The listing builds one solid part. Answer for the finished solid, in the listing's coordinates (mm). Face numbers are marked on the shaded views. A direction names the side the tool comes from. Coordinates: 2 decimals unless noted, no trailing zeros. Order: outer loops, then holes, each group sorted by start corner. A loop starts at its lowest first (then second) coordinate and runs counter-clockwise, first axis right, second up. Notation, with made-up numbers: (46, 13) -> (93, 13) arc R22 ccw to (93, 37) -> close; hole circle Ø5 at (25.25, -10.75). An arc over 180 degrees is marked (long way). Write each question's results on one line, items separated by ' | '. Start each with the question number.
(1) The part is cut by section D-D, the plane y = -47. Give the vertices of the cut face in (x, z), then the cut area to 3 significant figures.
(2) Determine the mould class of the marked faces 4, 5, 6 and 7 for opening direction Y: +Y half, -Y half, draft (parallel to the pull), parting line (faces both ways), or undercut.
(3) The part is cut by section B-B, the plane x = 73. Give the vertices of the cut face in (y, z), then the cut area to 3 significant figures.
(4) Given pin 1 (1.5 mm diameter, centred on x = 68, z = -24.5, fed in from +Y), flat-ended and moving along its own axis, determine where the tip first touches the part or whether it passes through.
(5) A tool of negligible diameter and unlimited length cuts with its end or side. For the marked faces 1, 2 and 3, from which of +Z, -Z, +X, -X, +Y, -Y can it reach the whole face along a straight path? Write none if from no direction.
(6) The part is cut by section A-A, the plane z = 17.5. Give the vertices of the cut face in (x, y).
(7) Straight lines are drawn through the part: L1, parallel to Y at x = -40.5, z = -9; L2, parallel to Y at x = -65, z = 15; L3, parallel to Z at x = 1, y = -57.5. For each, find the intervals that lie inside material, in ascending order.
(8) The part is cut by section C-C, the plane z = 2. Give the vertices of the cut face in (x, y), then the cut area to 3 significant figures.
```python
from build123d import *

# Parameters (mm, degrees)
F0_W      = 180.589676
F0_H      = 76.531302
F1_DEPTH  = 127
F4_DEPTH  = 127.001
F6_DEPTH  = 25.4
F8_DEPTH  = 25.4
F9_R      = 10.785345
F9_R_2    = 11.594885
F10_DEPTH = 25.4


with BuildPart() as f1:
    # F0 (on Front) → F1 (new body)
    with BuildSketch(Plane.XZ):
        with Locations((-1.058735, -6.049903)):
            Rectangle(F0_W, F0_H)
    extrude(amount=F1_DEPTH)

    # F2 (on face) → F4 (cut, through all)
    with BuildSketch(Plane.XZ.offset(127)):
        with BuildLine():
            Line((31.005763, 32.215748), (-31.913254, 32.215748))
            ThreePointArc((-31.913254, 32.215748), (-0.453746, 5.58325), (31.005763, 32.215748))
        make_face()
    extrude(amount=-F4_DEPTH, mode=Mode.SUBTRACT)

    # F3 (on face) → F6 (join)
    with BuildSketch(Plane.XZ.offset(127)):
        with BuildLine():
            ThreePointArc((31.005763, 32.215748), (-0.453746, 5.58325), (-31.913254, 32.215748))
            Line((-31.913254, 32.215748), (-40.383123, 32.215748))
            ThreePointArc((-40.383123, 32.215748), (-2e-06, -2.234087), (40.383119, 32.215748))
            Line((40.383119, 32.215748), (31.005763, 32.215748))
        make_face()
    extrude(amount=F6_DEPTH)

    # F7 (on face) → F8 (join)
    with BuildSketch(Plane(origin=(0, 0, 0), x_dir=(-1, 0, 0), z_dir=(0, 1, 0))):
        with BuildLine():
            Line((-31.005763, 32.215748), (-38.87064, 32.215748))
            ThreePointArc((-38.87064, 32.215748), (1.058737, -1.02799), (40.988114, 32.215748))
            Line((40.988114, 32.215748), (31.913254, 32.215748))
            ThreePointArc((31.913254, 32.215748), (0.453746, 5.58325), (-31.005763, 32.215748))
        make_face()
    extrude(amount=F8_DEPTH)

    # F9 (on face) → F10 (cut)
    with BuildSketch(Plane.XY.offset(32.215748)):
        with Locations((-63.675255, -62.828988)):
            Circle(F9_R)
        with Locations((64.280249, -62.828988)):
            Circle(F9_R_2)
    extrude(amount=-F10_DEPTH, mode=Mode.SUBTRACT)


solid = f1.part
```
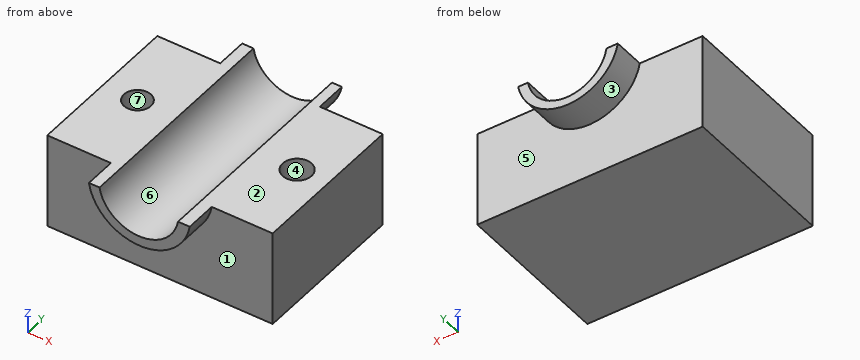
Established:
1) outline: (-91.35, -44.32) -> (89.24, -44.32) -> (89.24, 32.22) -> (31.01, 32.22) arc R31.9 cw to (-31.91, 32.22) -> (-91.35, 32.22) -> close | area: 12,600 mm^2
2) face 4: undercut | face 5: +Y half | face 6: draft | face 7: undercut
3) outline: (-127, -44.32) -> (0, -44.32) -> (0, 32.22) -> (-55.19, 32.22) -> (-55.19, 6.82) -> (-70.47, 6.82) -> (-70.47, 32.22) -> (-127, 32.22) -> close | area: 9,330 mm^2
4) pin 1: stops at y = 0
5) face 1: -Z, -Y | face 2: +Z, +X, -X, +Y, -Y | face 3: -Z, +Y
6) outline: (-91.35, -127) -> (-34.99, -127) -> (-34.99, -152.4) -> (-25.32, -152.4) -> (-25.32, 25.4) -> (-35.14, 25.4) -> (-35.14, 0) -> (-91.35, 0) -> close; (24.41, -152.4) -> (34.99, -152.4) -> (34.99, -127) -> (89.24, -127) -> (89.24, 0) -> (33.02, 0) -> (33.02, 25.4) -> (24.41, 25.4) -> close; hole circle Ø21.57 at (-63.68, -62.83); hole circle Ø23.19 at (64.28, -62.83)
7) L1: y = -127 to 0 | L2: y = -127 to -73.53, -52.13 to 0 | L3: z = -44.32 to 5.62
8) outline: (-91.35, -127) -> (-18.12, -127) -> (-18.12, -152.4) -> (18.12, -152.4) -> (18.12, -127) -> (89.24, -127) -> (89.24, 0) -> (14.33, 0) -> (14.33, 25.4) -> (-16.44, 25.4) -> (-16.44, 0) -> (-91.35, 0) -> close | area: 24,600 mm^2
